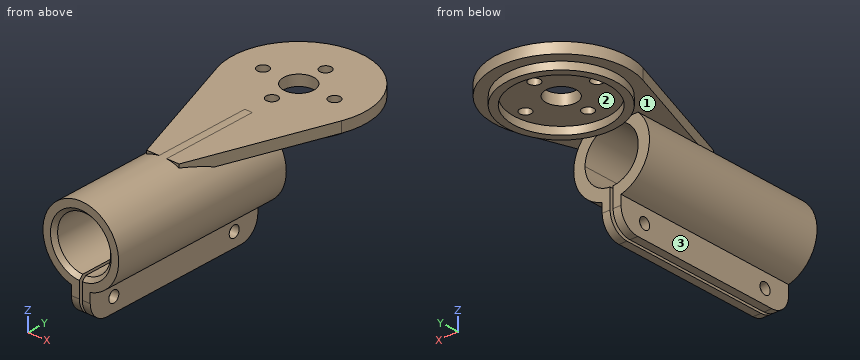
from build123d import *

# Parameters (mm, degrees)
F0_R      = 10.05
F0_R_2    = 7.05
F1_DEPTH  = 50
F3_R      = 17.5
F4_DEPTH  = 2.8
F5_W      = 5
F5_H      = 10
F6_DEPTH  = 50
F7_W      = 0.8
F7_H      = 12.637284
F8_DEPTH  = 82.538162
F10_DEPTH = 2.8
F11_R     = 1.5
F11_R_2   = 4
F12_DEPTH = 25
F13_R     = 14.5
F13_R_2   = 12.5
F14_DEPTH = 2
F15_R     = 1.5
F16_DEPTH = 20.001
F17_R     = 5
F18_SIZE  = 1


with BuildPart() as f1:
    # F0 (on Front) → F1 (new body)
    with BuildSketch(Plane.XZ):
        Circle(F0_R)
        Circle(F0_R_2, mode=Mode.SUBTRACT)
    extrude(amount=F1_DEPTH)

    # F3 (on offset) → F4 (join)
    with BuildSketch(Plane.XY.offset(10)):
        with Locations((0, 15.037162)):
            Circle(F3_R)
    extrude(amount=-F4_DEPTH)

    # F5 (on face) → F6 (join, through all)
    with BuildSketch(Plane.XZ.offset(50)):
        with Locations((0, -12.213485)):
            Rectangle(F5_W, F5_H)
    extrude(amount=-F6_DEPTH)

    # F7 (on face) → F8 (cut, through all)
    with BuildSketch(Plane.XZ.offset(50)):
        with Locations((0, -12.604385)):
            Rectangle(F7_W, F7_H)
    extrude(amount=-F8_DEPTH, mode=Mode.SUBTRACT)

    # F9 (on face) → F10 (join)
    with BuildSketch(Plane.XY.offset(10)):
        Polygon((4.304297, -25.528217), (16.511778, 9.239647), (-16.511778, 9.239647), (-4.315564, -25.528217), align=None)
    extrude(amount=-F10_DEPTH)

    # F11 (on face) → F12 (cut)
    with BuildSketch(Plane.XY.offset(10)):
        with Locations((0, 23.037162)):
            Circle(F11_R)
        with Locations((-9.5, 15.037162)):
            Circle(F11_R)
        with Locations((0, 7.037162)):
            Circle(F11_R)
        with Locations((9.5, 15.037162)):
            Circle(F11_R)
        with Locations((0, 15.037162)):
            Circle(F11_R_2)
    extrude(amount=-F12_DEPTH, mode=Mode.SUBTRACT)

    # F13 (on face) → F14 (join)
    with BuildSketch(Plane(origin=(0, 0, 7.2), x_dir=(1, 0, 0), z_dir=(0, 0, -1))):
        with Locations((0, -15.037162)):
            Circle(F13_R)
        with Locations((0, -15.037162)):
            Circle(F13_R_2, mode=Mode.SUBTRACT)
    extrude(amount=F14_DEPTH)

    # F15 (on face) → F16 (cut, through all)
    with BuildSketch(Plane.YZ.offset(2.5)):
        with Locations((-7.034952, -13.473787)):
            Circle(F15_R)
        with Locations((-42.965048, -13.473787)):
            Circle(F15_R)
    extrude(amount=-F16_DEPTH, mode=Mode.SUBTRACT)

    # F17
    f17_edges = [f1.edges().sort_by_distance(p)[0] for p in [
        (1.45, -50, -17.213485),
        (-1.45, -50, -17.213485),
        (1.45, 0, -17.213485),
        (-1.45, 0, -17.213485),
    ]]
    fillet(f17_edges, radius=F17_R)

    # F18
    f18_edges = [f1.edges().sort_by_distance(p)[0] for p in [
        (-4.841616, -50, 5.124573),
    ]]
    chamfer(f18_edges, length=F18_SIZE)


solid = f1.part
Could you check a few things on this model? Use its own coordinates, in mm. Face numbers are marked on the shaded views. Coordinates: 2 decimals unless noted, no trailing zeros. Order: outer loops, then holes, each group sorted by start corner. A loop starts at its lowest first (then second) coordinate and runs counter-clockwise, first axis right, second up.
Q1. Suppose I cut it at B-B on y = -15. Please give me the cut outline in (x, z).
Q2. Suppose I cut it at A-A on y = -32.5. Please give me the cut outline in (x, z), and give its area (3 significant figures).
Q3. Thinking about a two-plate mould opening in X: for the marked faces 1, 2 and 3, which applies, released by +X, released by -X, zero draft, split by the parting line, or undercut?
Q4. Please list where these lines run through material, in increasing order: L1, parallel to Y at x = 0, z = 6.15; L2, parallel to X at y = -39.5, z = 0.5; L3, parallel to X at y = -37.5, z = -9.75.
Q5. Suppose I cut it at C-C on y = 20.5. Please give me the cut outline in (x, z).
Q6. Will these pins go through, and if not, where does the flat tip stop? pin 1 (5 mm diameter, centred on y = -7.03, z = -13.47, fed in from +X); pin 2 (5 mm diameter, centred on x = -9.5, y = 15.04, fed in from +Z); pin 3 (3 mm diameter, centred on x = -9.5, y = 4, fed in from -Z); pin 4 (6 mm diameter, centred on x = -13, z = 0.5, fed in from -Y).
Answer:
1. outline: (-8.01, 7.2) - (-7.01, 7.2) arc R10.05 ccw to (-2.5, -9.73) - (-2.5, -17.21) - (-0.4, -17.21) - (-0.4, -7.04) arc R7.05 cw (long way) to (0.4, -7.04) - (0.4, -17.21) - (2.5, -17.21) - (2.5, -9.73) arc R10.05 ccw to (7.01, 7.2) - (8, 7.2) - (8, 10) - (1, 10) arc R10.05 ccw to (-1, 10) - (-8.01, 10) - close
2. outline: (-2.5, -17.21) - (-0.4, -17.21) - (-0.4, -7.04) arc R7.05 cw (long way) to (0.4, -7.04) - (0.4, -17.21) - (2.5, -17.21) - (2.5, -9.73) arc R10.05 ccw (long way) to (-2.5, -9.73) - close
2. area: 189 mm2
3. face 1: zero draft
3. face 2: undercut
3. face 3: released by -X
4. L1: y = 0.54 to 2.54, 27.54 to 29.54
4. L2: x = -10.04 to -7.03, 7.03 to 10.04
4. L3: x = -2.5 to -0.4, 0.4 to 2.5
5. outline: (-16.63, 7.2) - (-13.43, 7.2) - (-13.43, 5.2) - (-11.24, 5.2) - (-11.24, 7.2) - (11.24, 7.2) - (11.24, 5.2) - (13.43, 5.2) - (13.43, 7.2) - (16.63, 7.2) - (16.63, 10) - (-16.63, 10) - close
6. pin 1: stops at x = 2.5
6. pin 2: stops at z = 10
6. pin 3: stops at z = 5.2
6. pin 4: stops at y = -50
